Design review of the part shown in the three views and the two pictorial views. Dimensions are in mm from the part's minimum x, y and z. A direction names the side the tool comes from. Give positions to 0.01 mm unless a question says otherwise; leave off trailing zeros. Loops run counter-clockwise (first coordinate to the right, second up) from the corner with the lowest first, then second, coordinate; pieces in that order, holes last. Notation, with made-up numbers: (38.25, -11.5) - (71.25, -11.5) arc R26 ccw to (71.25, 5.5) - close; hole circle Ø2 at (34, 2.5). An arc over 180 degrees is marked (long way). Answer as a JSON object with one key per item and string values.
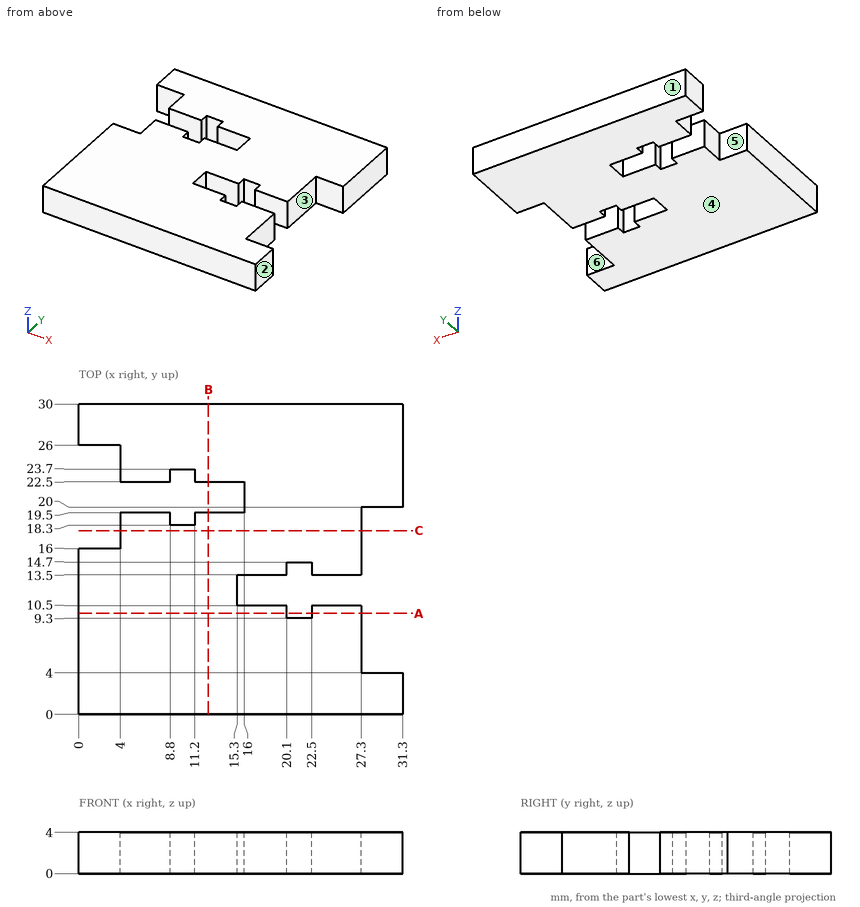
Q1. The part is to be moulded in two halves that separate along Y. For the marked faces 1, 2 and 3, say which applies: +Y half, -Y half, draft (parallel to the pull), parting line (faces both ways), or undercut.
Results:
{"face 1": "+Y half", "face 2": "draft", "face 3": "undercut"}
Q2. For the marked faces 4, 5 and 6, list the 3-axis set-ups (+Z, -Z, +X, -X, +Y, -Y) from which the entire face can be reached by the end or side of a thin tool; tool diameter is ignored.
Results:
{"face 4": "-Z, +X, -X, +Y, -Y", "face 5": "+Z, -Z, -X", "face 6": "+Z, -Z, +X"}
Q3. Consider section A-A, the plane y = 9.75. State the section outline as (x, z) points, plus the area to 3 significant figures.
Results:
{"outline": "(0, 0) - (20.1, 0) - (20.1, 4) - (0, 4) - close; (22.5, 0) - (27.3, 0) - (27.3, 4) - (22.5, 4) - close", "area": "99.6 mm^2"}
Q4. To check wall thickness, follow probe 1 along Y at (x, z) = (21, 0.55); probe 2 along Y at (x, z) = (2, 2.5); probe 3 along X at (y, z) = (19.25, 1.55). State the ranges of each line that lie inside material, in increasing order. Write a range as [from, to].
Results:
{"probe 1": "y = [0, 9.3], [14.7, 30]", "probe 2": "y = [0, 16], [26, 30]", "probe 3": "x = [4, 8.8], [11.2, 27.3]"}
Q5. Clearance check with flat-ended pins moving along their axes: pin 1 Ø10 at (x, y) = (13.5, 24.5) entering from -Z; pin 2 Ø1.5 at (y, z) = (23.5, 1.5) entering from -X. State where each tip first meets the part, or that it passes through.
Results:
{"pin 1": "stops at z = 0", "pin 2": "stops at x = 4"}
Q6. Consider section C-C, the plane y = 17.75. State the section outline as (x, z) points.
Results:
{"outline": "(4, 0) - (27.3, 0) - (27.3, 4) - (4, 4) - close"}
Q7. Consider section B-B, the plane x = 12.5. State the section outline as (y, z) points, plus the area to 3 significant figures.
Results:
{"outline": "(0, 0) - (19.5, 0) - (19.5, 4) - (0, 4) - close; (22.5, 0) - (30, 0) - (30, 4) - (22.5, 4) - close", "area": "108 mm^2"}
